Part model, mm, in its own coordinate system. A direction names the side the tool comes from. Coordinates: 2 decimals unless noted, no trailing zeros. Write each loop counter-clockwise with the first axis right and the second up, starting at its lowest first coordinate (ties: lowest second). Pieces come first, ordered by that corner, then holes. Notation, with made-up numbers: (-38.5, 24.25) -> (2.5, 24.25) arc R28 ccw to (2.5, 51.25) -> close; hole circle Ø9 at (63.5, -11.75). An arc over 180 degrees is marked (long way). Write item = value, one per line. Start each with the question number.
Q1. Pin check, flat tips, straight feed: P1, Ø3.5, axis at y = 0, z = 108, coming from the +X side; P2, Ø6.5, axis at x = -35, y = 7, coming from the -Z side; P3, Ø6.5, axis at x = -50.5, y = -6, coming from the -Z side. Stop position of each tip, or through.
Q2. Band-saw the part on B-B, the plane x = -23. List the corners of the cut face in (y, z), plus the area to 3 significant figures.
Q3. Tool access for faces 5 (the cylindrical face through (-69.94, -0.65, 105.07)), 6 (the flat face through (-41, -7, 96)), 7 (the flat face through (-41, 7, 96)): list every direction of +Z, -Z, +X, -X, +Y, -Y with a clear straight run to the whole face (end or side of a thin tool).
Q4. Pull direction Y, two halves, no side cores. Call faces 1 (the conical face through (-39.54, 0.05, 111.02)), 2 (the flat face through (-74, 0, 103)), 3 (the cylindrical face through (-44.04, -2.3, 119.92)), 4 (the flat face through (-36, 10, 111)): released by +Y, released by -Y, zero draft, split by the parting line, or undercut.
Q5. Probe line 1 (Y direction, x = -38.5, z = 117.75); line 2 (Z direction, x = -72, y = 0); line 3 (X direction, y = 0, z = 121.75). List the from-to ranges inside material, lowest first.
Q6. Band-saw the part on D-D, the plane x = -33.5. Give the number of separate pieces and of enclosed holes in the cut face, plus the area to 3 significant figures.
Q7. Band-saw the part on C-C, the plane z = 121. List the corners of the cut face in (x, y).
Q8. Band-saw the part on A-A, the plane x = -68.5. List the corners of the cut face in (y, z).
from build123d import *

# Parameters (mm, degrees)
F1_DEPTH     = 11.5
F3_DEPTH     = 5
F5_D         = 14
F5_DEPTH     = 36
F5_TIP       = 4.2060243332
F7_D         = 6.8
F7_DEPTH     = 17
F7_TIP       = 2.0429261047
F8_SIZE2     = 9.237604307
F8_SIZE      = 16
F8_2_SIZE2   = 9.237604307
F8_2_SIZE    = 16
F9_T1_DEPTH  = 23
F9_T6_DEPTH  = 84.5247913859
F9_T12_DEPTH = 98.4752086141
F9_T18_DEPTH = 98.4752086141
F9_T25_DEPTH = 98.4752086141
F9_T32_DEPTH = 98.4752086141
F9_T38_DEPTH = 98.4752086141
F9_T44_DEPTH = 98.4752086141
F9_T51_DEPTH = 98.4752086141
F9_T58_DEPTH = 98.4752086141
F11_DEPTH    = 74
F13_DEPTH    = 20
F14_SIZE2    = 10
F14_SIZE     = 10
F16_D        = 12
F16_DEPTH    = 12
F16_TIP      = 3.6051637142
F17_R        = 2
F18_DEPTH    = 20
F21_D        = 6
F21_DEPTH    = 8
F21_TIP      = 1.8025818571


# Not quite as in the source:
# - a fillet or chamfer that OpenCascade refuses, or shapes differently, is made with other operations: its cross-section is extruded or revolved along the edge and cut away or added


with BuildPart() as f1:
    # F0 (on Front) → F1 (new body, symmetric)
    with BuildSketch(Plane.XZ):
        Polygon((-200, 0), (0, 0), (0, 40), (-63, 40), (-63, 155), (0, 155), (0, 185), (-90, 185), (-200, 30), align=None)
    extrude(amount=F1_DEPTH, both=True)

    # F2 (on face) → F3 (cut)
    with BuildSketch(Plane.YZ.offset(-63)):
        with BuildLine():
            ThreePointArc((3.5, 135), (0, 138.5), (-3.5, 135))
            Line((-3.5, 135), (-3.5, 67))
            ThreePointArc((-3.5, 67), (0, 63.5), (3.5, 67))
            Line((3.5, 67), (3.5, 135))
        make_face()
    extrude(amount=-F3_DEPTH, mode=Mode.SUBTRACT)

    # F5
    with Locations(Plane.XY.offset(185)):
        with Locations((-20, 0)):
            Hole(F5_D / 2, depth=F5_DEPTH)
            with Locations((0, 0, -(F5_DEPTH + F5_TIP / 2))):  # 118° drill point
                Cone(0, F5_D / 2, F5_TIP, mode=Mode.SUBTRACT)

    # F7
    with Locations(Plane(origin=(0, 0, 0), x_dir=(1, 0, 0), z_dir=(0, 0, -1))):
        with Locations((-175, 0), (-125, 0), (-75, 0), (-25, 0)):
            Hole(F7_D / 2, depth=F7_DEPTH)
            with Locations((0, 0, -(F7_DEPTH + F7_TIP / 2))):  # 118° drill point
                Cone(0, F7_D / 2, F7_TIP, mode=Mode.SUBTRACT)

    # F8
    f8_edges = [f1.edges().sort_by_distance(p)[0] for p in [
        (-31.5, -11.5, 40),
    ]]
    f8_side = f1.faces().sort_by_distance((-97.944693, -11.5, 74.396883))[0]
    chamfer(f8_edges, length=F8_SIZE, length2=F8_SIZE2, reference=f8_side)

    # F8#2
    f8_2_edges = [f1.edges().sort_by_distance(p)[0] for p in [
        (-31.5, 11.5, 40),
    ]]
    f8_2_side = f1.faces().sort_by_distance((-97.944693, 11.5, 74.396883))[0]
    chamfer(f8_2_edges, length=F8_2_SIZE, length2=F8_2_SIZE2, reference=f8_2_side)

    # F9: fillet of radius 16 on 4 edges, made by hand

    # F9_s2 → F9_t1 (join)
    with BuildSketch(Plane.XZ.offset(-11.5)):
        with BuildLine():
            ThreePointArc((-63, 139), (-58.313708499, 150.313708499), (-47, 155))
            Line((-47, 155), (-63, 155))
            Line((-63, 155), (-63, 139))
        make_face()
    extrude(amount=F9_T1_DEPTH)


with BuildPart() as f9_tool4:
    # F9_s5 → F9_t6 (new body)
    with BuildSketch(Plane.XZ.offset(-42.262395693)):
        with BuildLine():
            ThreePointArc((-47, 40), (-58.313708499, 44.686291501), (-63, 56))
            Line((-63, 56), (-63, 40))
            Line((-63, 40), (-47, 40))
        make_face()
    extrude(amount=F9_T6_DEPTH)

    split(bisect_by=Plane.XZ.offset(-11.5), keep=Keep.TOP)

    split(bisect_by=Plane.XZ.offset(11.5), keep=Keep.BOTTOM)


with BuildPart() as f1_1:
    add(f1.part)

    # F9_t3: union F9_tool4
    add(f9_tool4.part)


with BuildPart() as f9_tool10:
    # F9_s11 → F9_t12 (new body)
    with BuildSketch(Plane(origin=(0, -12.4826951546, -21.6206622231), x_dir=(1, 0, 0), z_dir=(0, 0.5, 0.8660254038))):
        with BuildLine():
            ThreePointArc((-47, -21.9592921435), (-58.313708499, -26.6455836445), (-63, -37.9592921435))
            Line((-63, -37.9592921435), (-63, -21.9592921435))
            Line((-63, -21.9592921435), (-47, -21.9592921435))
        make_face()
    extrude(amount=F9_T12_DEPTH)

    split(bisect_by=Plane.XY.offset(40), keep=Keep.BOTTOM)

    split(bisect_by=Plane.XZ.offset(11.5), keep=Keep.TOP)


with BuildPart() as f1_2:
    add(f1_1.part)

    # F9_t9: union F9_tool10
    add(f9_tool10.part)


with BuildPart() as f9_tool16:
    # F9_s17 → F9_t18 (new body)
    with BuildSketch(Plane(origin=(0, -12.4826951546, -21.6206622231), x_dir=(1, 0, 0), z_dir=(0, 0.5, 0.8660254038))):
        with BuildLine():
            ThreePointArc((-47, -21.9592921435), (-58.313708499, -26.6455836445), (-63, -37.9592921435))
            Line((-63, -37.9592921435), (-63, -21.9592921435))
            Line((-63, -21.9592921435), (-47, -21.9592921435))
        make_face()
    extrude(amount=F9_T18_DEPTH)

    split(bisect_by=Plane.XY.offset(40), keep=Keep.BOTTOM)

    split(bisect_by=Plane.XZ.offset(11.5), keep=Keep.BOTTOM)

    split(bisect_by=Plane.XZ.offset(3.5), keep=Keep.TOP)


with BuildPart() as f1_3:
    add(f1_2.part)

    # F9_t15: union F9_tool16
    add(f9_tool16.part)


with BuildPart() as f9_tool23:
    # F9_s24 → F9_t25 (new body)
    with BuildSketch(Plane(origin=(0, -12.4826951546, -21.6206622231), x_dir=(1, 0, 0), z_dir=(0, 0.5, 0.8660254038))):
        with BuildLine():
            ThreePointArc((-47, -21.9592921435), (-58.313708499, -26.6455836445), (-63, -37.9592921435))
            Line((-63, -37.9592921435), (-63, -21.9592921435))
            Line((-63, -21.9592921435), (-47, -21.9592921435))
        make_face()
    extrude(amount=F9_T25_DEPTH)

    split(bisect_by=Plane.XY.offset(40), keep=Keep.TOP)

    split(bisect_by=Plane.XZ.offset(11.5), keep=Keep.BOTTOM)

    split(bisect_by=Plane.XZ.offset(3.5), keep=Keep.TOP)


with BuildPart() as f1_4:
    add(f1_3.part)

    # F9_t22: union F9_tool23
    add(f9_tool23.part)


with BuildPart() as f9_tool30:
    # F9_s31 → F9_t32 (new body)
    with BuildSketch(Plane(origin=(0, -12.4826951546, -21.6206622231), x_dir=(1, 0, 0), z_dir=(0, 0.5, 0.8660254038))):
        with BuildLine():
            ThreePointArc((-47, -21.9592921435), (-58.313708499, -26.6455836445), (-63, -37.9592921435))
            Line((-63, -37.9592921435), (-63, -21.9592921435))
            Line((-63, -21.9592921435), (-47, -21.9592921435))
        make_face()
    extrude(amount=F9_T32_DEPTH)

    split(bisect_by=Plane.XY.offset(40), keep=Keep.BOTTOM)

    split(bisect_by=Plane.XZ.offset(3.5), keep=Keep.BOTTOM)


with BuildPart() as f1_5:
    add(f1_4.part)

    # F9_t29: union F9_tool30
    add(f9_tool30.part)


with BuildPart() as f9_tool36:
    # F9_s37 → F9_t38 (new body)
    with BuildSketch(Plane(origin=(0, 12.4826951546, -21.6206622231), x_dir=(1, 0, 0), z_dir=(0, -0.5, 0.8660254038))):
        with BuildLine():
            ThreePointArc((-47, 21.9592921435), (-58.313708499, 26.6455836445), (-63, 37.9592921435))
            Line((-63, 37.9592921435), (-63, 21.9592921435))
            Line((-63, 21.9592921435), (-47, 21.9592921435))
        make_face()
    extrude(amount=F9_T38_DEPTH)

    split(bisect_by=Plane.XY.offset(40), keep=Keep.BOTTOM)

    split(bisect_by=Plane.XZ.offset(-11.5), keep=Keep.BOTTOM)


with BuildPart() as f1_6:
    add(f1_5.part)

    # F9_t35: union F9_tool36
    add(f9_tool36.part)


with BuildPart() as f9_tool42:
    # F9_s43 → F9_t44 (new body)
    with BuildSketch(Plane(origin=(0, 12.4826951546, -21.6206622231), x_dir=(1, 0, 0), z_dir=(0, -0.5, 0.8660254038))):
        with BuildLine():
            ThreePointArc((-47, 21.9592921435), (-58.313708499, 26.6455836445), (-63, 37.9592921435))
            Line((-63, 37.9592921435), (-63, 21.9592921435))
            Line((-63, 21.9592921435), (-47, 21.9592921435))
        make_face()
    extrude(amount=F9_T44_DEPTH)

    split(bisect_by=Plane.XY.offset(40), keep=Keep.BOTTOM)

    split(bisect_by=Plane.XZ.offset(-11.5), keep=Keep.TOP)

    split(bisect_by=Plane.XZ.offset(-3.5), keep=Keep.BOTTOM)


with BuildPart() as f1_7:
    add(f1_6.part)

    # F9_t41: union F9_tool42
    add(f9_tool42.part)


with BuildPart() as f9_tool49:
    # F9_s50 → F9_t51 (new body)
    with BuildSketch(Plane(origin=(0, 12.4826951546, -21.6206622231), x_dir=(1, 0, 0), z_dir=(0, -0.5, 0.8660254038))):
        with BuildLine():
            ThreePointArc((-47, 21.9592921435), (-58.313708499, 26.6455836445), (-63, 37.9592921435))
            Line((-63, 37.9592921435), (-63, 21.9592921435))
            Line((-63, 21.9592921435), (-47, 21.9592921435))
        make_face()
    extrude(amount=F9_T51_DEPTH)

    split(bisect_by=Plane.XY.offset(40), keep=Keep.TOP)

    split(bisect_by=Plane.XZ.offset(-11.5), keep=Keep.TOP)

    split(bisect_by=Plane.XZ.offset(-3.5), keep=Keep.BOTTOM)


with BuildPart() as f1_8:
    add(f1_7.part)

    # F9_t48: union F9_tool49
    add(f9_tool49.part)


with BuildPart() as f9_tool56:
    # F9_s57 → F9_t58 (new body)
    with BuildSketch(Plane(origin=(0, 12.4826951546, -21.6206622231), x_dir=(1, 0, 0), z_dir=(0, -0.5, 0.8660254038))):
        with BuildLine():
            ThreePointArc((-47, 21.9592921435), (-58.313708499, 26.6455836445), (-63, 37.9592921435))
            Line((-63, 37.9592921435), (-63, 21.9592921435))
            Line((-63, 21.9592921435), (-47, 21.9592921435))
        make_face()
    extrude(amount=F9_T58_DEPTH)

    split(bisect_by=Plane.XY.offset(40), keep=Keep.BOTTOM)

    split(bisect_by=Plane.XZ.offset(-3.5), keep=Keep.TOP)


with BuildPart() as f1_9:
    add(f1_8.part)

    # F9_t55: union F9_tool56
    add(f9_tool56.part)


with BuildPart() as f11:
    # F10 (on Right) → F11 (new body)
    with BuildSketch(Plane.YZ):
        Polygon((-2, 90), (0, 90), (2, 90), (4.3, 95.5526911935), (4.3, 96), (10, 96), (10, 126), (0, 126), (-10, 126), (-10, 96), (-4.3, 96), (-4.3, 95.5526911935), align=None)
    extrude(amount=-F11_DEPTH)

    # F12 (on face) → F13 (cut, through all)
    with BuildSketch(Plane.XZ.offset(10)):
        Polygon((0, 90), (0, 111), (-12.124355653, 90), align=None)
    extrude(amount=-F13_DEPTH, mode=Mode.SUBTRACT)

    # F14
    f14_edges = [f11.edges().sort_by_distance(p)[0] for p in [
        (-74, 0, 126),
    ]]
    chamfer(f14_edges, length=F14_SIZE, length2=F14_SIZE2)

    # F16
    with Locations(Plane.XY.offset(126)):
        with Locations((-38.5, 0)):
            Hole(F16_D / 2, depth=F16_DEPTH)
            with Locations((0, 0, -(F16_DEPTH + F16_TIP / 2))):  # 118° drill point
                Cone(0, F16_D / 2, F16_TIP, mode=Mode.SUBTRACT)

    # F17 (on face) → F18 (cut, through all)
    with BuildSketch(Plane.XZ.offset(10)):
        with Locations((-33.5, 121)):
            Circle(F17_R)
    extrude(amount=-F18_DEPTH, mode=Mode.SUBTRACT)

    # F21
    with Locations(Plane(origin=(-74, 0, 0), x_dir=(0, -1, 0), z_dir=(-1, 0, 0))):
        with Locations((0, 108)):
            Hole(F21_D / 2, depth=F21_DEPTH)
            with Locations((0, 0, -(F21_DEPTH + F21_TIP / 2))):  # 118° drill point
                Cone(0, F21_D / 2, F21_TIP, mode=Mode.SUBTRACT)


solid = f11.part
Ans:
q1.P1 = -0.72
q1.P2 = 94.22
q1.P3 = 91.81
q2.outline = (-10, 96) -> (-4.3, 96) -> (-4.3, 95.55) -> (-2, 90) -> (2, 90) -> (4.3, 95.55) -> (4.3, 96) -> (10, 96) -> (10, 126) -> (-10, 126) -> close
q2.area = 639 mm2
q3.face_5 = -X
q3.face_6 = -Z, +X, -X, -Y
q3.face_7 = -Z, +X, -X, +Y
q4.face_1 = undercut
q4.face_2 = zero draft
q4.face_3 = undercut
q4.face_4 = released by +Y
q5.line_1 = -10 to -6, 6 to 10
q5.line_2 = 90 to 105, 111 to 118
q5.line_3 = -68.25 to -44.5, -31.65 to 0
q6.separate_pieces = 3
q6.enclosed_holes = 0
q6.area = 503 mm2
q7.outline = (-69, -10) -> (-35.5, -10) -> (-35.5, -5.2) arc R6 cw (long way) to (-35.5, 5.2) -> (-35.5, 10) -> (-69, 10) -> close; (-31.5, -10) -> (0, -10) -> (0, 10) -> (-31.5, 10) -> close
q8.outline = (-10, 96) -> (-4.3, 96) -> (-4.3, 95.55) -> (-2, 90) -> (2, 90) -> (4.3, 95.55) -> (4.3, 96) -> (10, 96) -> (10, 121.5) -> (-10, 121.5) -> close; hole circle Ø6 at (0, 108)
